Could you check a few things on this model? Use its own coordinates, in mm. Face numbers are marked on the shaded views. A direction names the side the tool comes from. Round coordinates to 2 decimals unless told otherwise and drop trailing zeros. Order: outer loops, then holes, each group sorted by start corner. A loop starts at its lowest first (then second) coordinate and runs counter-clockwise, first axis right, second up. Notation, with made-up numbers: (39.25, 58) -> (45.25, 58) arc R8 ccw to (45.25, 62) -> close; hole circle Ø7 at (24, 42.5). An arc over 180 degrees is marked (long way). Put each result on its own line as item: value. Start each with the question number.
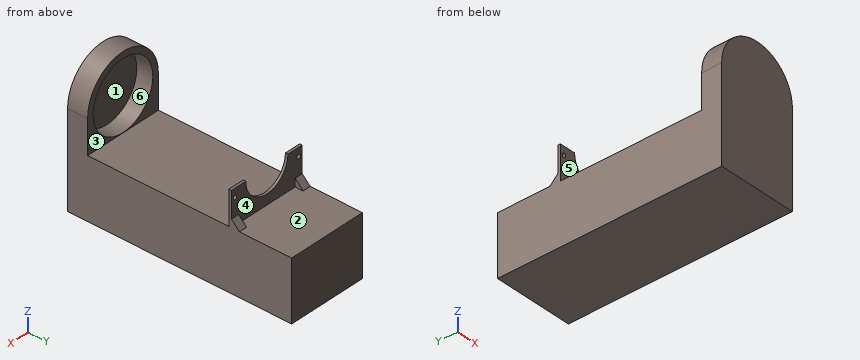
from build123d import *

# Parameters (mm, degrees)
SKETCH1_W            = 50.8
SKETCH1_H            = 142.24
BOSS_EXTRUDE1_DEPTH  = 38.1
SKETCH8_R            = 21.43125
BOSS_EXTRUDE2_DEPTH  = 2.54
SKETCH8_5_R          = 21.43125
BOSS_EXTRUDE9_DEPTH  = 12.7
BOSS_EXTRUDE13_DEPTH = 0.798558565
SKETCH16_R           = 1.27
CUT_EXTRUDE7_DEPTH   = 1.59711713
BOSS_EXTRUDE14_DEPTH = 5.08


with BuildPart() as part:
    # Sketch1 → Boss-Extrude1 (new body)
    with BuildSketch(Plane.XY):
        Rectangle(SKETCH1_W, SKETCH1_H)
    extrude(amount=BOSS_EXTRUDE1_DEPTH)



with BuildPart() as body_2:
    # Sketch8 → Boss-Extrude2 (new body)
    # profile 1 of 2: a face of its own
    with BuildSketch(Plane.XZ.offset(71.12)):
        with BuildLine():
            Line((-25.4, 38.1), (25.4, 38.1))
            Line((25.4, 38.1), (25.4, 59.69))
            ThreePointArc((25.4, 59.69), (0, 85.09), (-25.4, 59.69))
            Line((-25.4, 59.69), (-25.4, 38.1))
        make_face()
        with Locations((0, 59.69)):
            Circle(SKETCH8_R, mode=Mode.SUBTRACT)
    # profile 2 of 2: a face of its own
    with BuildSketch(Plane.XZ.offset(71.12)):
        with Locations((0, 59.69)):
            Circle(SKETCH8_R)
    extrude(amount=-BOSS_EXTRUDE2_DEPTH)


with BuildPart() as part_1:
    add(part.part)

    add(body_2.part)  # Boss-Extrude9 merges body 2
    # Sketch8<5> → Boss-Extrude9 (add)
    with BuildSketch(Plane.XZ.offset(71.12)):
        with BuildLine():
            Line((25.4, 38.1), (25.4, 59.69))
            ThreePointArc((25.4, 59.69), (0, 85.09), (-25.4, 59.69))
            Line((-25.4, 59.69), (-25.4, 38.1))
            Line((-25.4, 38.1), (25.4, 38.1))
        make_face()
        with Locations(Location((0, 59.69, 0), (0, 0, 270))):
            Circle(SKETCH8_5_R, mode=Mode.SUBTRACT)
    extrude(amount=-BOSS_EXTRUDE9_DEPTH)

    # Sketch15 → Boss-Extrude13 (add, symmetric)
    with BuildSketch(Plane(origin=(0, 32.108355434, 0), x_dir=(1, 0, 0), z_dir=(0, 1, 0))):
        with BuildLine():
            Line((-15.113, -59.69), (-25.4, -59.69))
            Line((-25.4, -59.69), (-25.4, -38.1))
            Line((-25.4, -38.1), (25.4, -38.1))
            Line((25.4, -38.1), (25.4, -59.69))
            Line((25.4, -59.69), (15.113, -59.69))
            ThreePointArc((15.113, -59.69), (0, -44.577), (-15.113, -59.69))
        make_face()
    extrude(amount=BOSS_EXTRUDE13_DEPTH, both=True)

    # Sketch16 → Cut-Extrude7 (cut)
    with BuildSketch(Plane(origin=(0, 32.906913999, 0), x_dir=(1, 0, 0), z_dir=(0, 1, 0))):
        with Locations(Location((-22.86, -54.356, 0), (0, 0, 270))):
            Circle(SKETCH16_R)
    cut_extrude7 = extrude(amount=-CUT_EXTRUDE7_DEPTH, mode=Mode.SUBTRACT)

    # Mirror1: Cut-Extrude7 across plane
    add(cut_extrude7.mirror(Plane(origin=(0, 0, 0), x_dir=(0, 0, 1), z_dir=(1, 0, 0))), mode=Mode.SUBTRACT)

    # Sketch17 → Boss-Extrude14 (add)
    with BuildSketch(Plane(origin=(25.4, 0, 0), x_dir=(0, 0, -1), z_dir=(1, 0, 0))):
        Polygon((-38.1, 32.906913999), (-38.1, 37.986913999), (-43.18, 32.906913999), align=None)
    boss_extrude14 = extrude(amount=-BOSS_EXTRUDE14_DEPTH)

    # Mirror2: Boss-Extrude14 across plane
    add(boss_extrude14.mirror(Plane(origin=(0, 0, 0), x_dir=(0, 0, 1), z_dir=(1, 0, 0))))


solid = part_1.part
1. Which directions (+Z, -Z, +X, -X, +Y, -Y) give clear straight access to the entire face, cutting with the end or side of a thin tool? Please do the marked faces 4, 5 and 6.
2. If we section it at A-A, the plane z = 50: Please give me the cut outline in (x, y).
3. I need wall thicknesses on L1, parallel to X at y = -62, z = 59; L2, parallel to Z at x = 22.86, y = 32.6; L3, parallel to Y at x = -3.5, z = 69. Which ranges of each line are inside material? Lowest first, please.
4. If we section it at C-C, the plane y = 57.5: Please give me the cut outline in (x, z), then the cut area to 3 significant figures.
5. Thinking about a two-plate mould opening in Z: for the marked faces 1, 2 and 3, which applies, +Z half, -Z half, draft (parallel to the pull), parting line (faces both ways), or undercut?
6. If we section it at B-B, the plane x = 0: Please give me the cut outline in (y, z).
7. For pin 1 Ø14 at (x, z) = (-9.5, 58.5) entering from +Y; pin 2 Ø1.3 at (x, y) = (-22, 32) entering from +Z; pin 3 Ø8 at (x, y) = (8.5, 18) entering from +Z; pin 4 Ø12 at (y, z) = (24, 63) entering from -X, each with a flat end and sliding along its axis, tell me the tip position at first contact or that it passes through.
Results below:
1. face 4: +Z, +Y
1. face 5: +Z, +X, -X
1. face 6: none
2. outline: (-25.4, -71.12) -> (25.4, -71.12) -> (25.4, -58.42) -> (19.12, -58.42) -> (19.12, -68.58) -> (-19.12, -68.58) -> (-19.12, -58.42) -> (-25.4, -58.42) -> close; (-25.4, 31.31) -> (-11.6, 31.31) -> (-11.6, 32.91) -> (-25.4, 32.91) -> close; (11.6, 31.31) -> (25.4, 31.31) -> (25.4, 32.91) -> (11.6, 32.91) -> close
3. L1: -25.4 to -21.42, 21.42 to 25.4
3. L2: 0 to 53.09, 55.63 to 59.69
3. L3: -71.12 to -68.58
4. outline: (-25.4, 0) -> (25.4, 0) -> (25.4, 38.1) -> (-25.4, 38.1) -> close
4. area: 1,940 mm2
5. face 1: undercut
5. face 2: +Z half
5. face 3: draft
6. outline: (-71.12, 0) -> (71.12, 0) -> (71.12, 38.1) -> (32.91, 38.1) -> (32.91, 44.58) -> (31.31, 44.58) -> (31.31, 38.1) -> (-58.42, 38.1) -> (-58.42, 38.26) -> (-68.58, 38.26) -> (-68.58, 81.12) -> (-58.42, 81.12) -> (-58.42, 85.09) -> (-71.12, 85.09) -> close
7. pin 1: y = 32.91
7. pin 2: z = 59.69
7. pin 3: z = 38.1
7. pin 4: through
